The listing builds one solid part. Answer for the finished solid, in the listing's coordinates (mm). A direction names the side the tool comes from. Give positions to 0.01 mm unless a question says otherwise; leave off trailing zeros. Order: outer loops, then holes, each group sorted by start corner. A loop starts at its lowest first (then second) coordinate and runs counter-clockwise, first axis right, second up. Notation, with made-up numbers: (-39, -36.5) - (-24, -36.5) arc R4 ccw to (-24, -30.5) - close; hole circle Ø11 at (88, 36.25). An arc over 180 degrees is marked (long way). Use a Markdown table: item, result. Add a question column.
1) Flat-ended cylindrical pins translate along their axes: pin 1 (4 mm diameter, centred on x = 182, z = -41.5, fed in from +Y); pin 2 (10.5 mm diameter, centred on y = 1, z = -3.5, fed in from -X); pin 3 (1 mm diameter, centred on x = 128, y = 26, fed in from -Z); pin 4 (10 mm diameter, centred on x = 170, y = 12, fed in from -Z). Find the tip coordinate at first contact, or state that the pin passes through.
2) Straight lines are drawn through the part: line 1 (X direction, y = 0.5, z = -5); line 2 (X direction, y = 8, z = -32.5); line 3 (Y direction, x = 50.5, z = -25). For each, find the intervals that lie inside material, in ascending order.
3) For faces 1 (the face through (55, 4, -4)), 2 (the face through (94.33, 14.79, -55.07)), 3 (the face through (148, 30, -10)), determine the directions among +Z, -Z, +X, -X, +Y, -Y from which every point of the face is accessible in a straight line to the end or side of a thin tool.
4) The mould has two halves that part along X. Classify faces 4 (the face through (150.07, 10.872, -4.832)), 5 (the face through (0, 13, -30)), 6 (the face through (149, 0, -41)), 7 (the face through (148, 17, 0)): released by +X, released by -X, zero draft, split by the parting line, or undercut.
5) Find section D-D, the plane z = -14. Determine the outline of the cut face in (x, y).
6) Find section B-B, the plane x = 50. Determine the outline of the cut face in (y, z), plus the area to 3 significant figures.
7) Find section C-C, the plane z = -43. Determine the outline of the cut face in (x, y).
8) Find section A-A, the plane y = 22. Determine the outline of the cut face in (x, z), plus the area to 3 significant figures.
from build123d import *

# Parameters (mm, degrees)
BOSS_EXTRU_1_DEPTH         = 30
ESQUISSE2_W                = 300
ESQUISSE2_H                = 60
BOSS_EXTRU_2_DEPTH         = 5
ESQUISSE3_W                = 10
ESQUISSE3_H                = 5.78
ENL_V_MAT_EXTRU_3_DEPTH    = 14.49
ESQUISSE5_W                = 10
ESQUISSE5_H                = 17.8
ENL_V_MAT_EXTRU_5_DEPTH    = 5
BOSS_EXTRU_4_REACH         = 256.018
ENL_V_MAT_EXTRU_6_DEPTH    = 10
R_P_TITION_LIN_AIRE1_COUNT = 3
R_P_TITION_LIN_AIRE1_PITCH = 100


with BuildPart() as part:
    # Esquisse1 → Boss.-Extru.1 (new body)
    with BuildSketch(Plane(origin=(0, 0, 0), x_dir=(1, 0, 0), z_dir=(0, 1, 0))):
        with BuildLine():
            Line((0, 0), (300, 0))
            Line((300, 0), (300, 60))
            Line((300, 60), (288.5, 50))
            ThreePointArc((288.5, 50), (250, 11.5), (211.5, 50))
            Line((211.5, 50), (200, 60))
            Line((200, 60), (188.5, 50))
            ThreePointArc((188.5, 50), (150, 11.5), (111.5, 50))
            Line((111.5, 50), (100, 60))
            Line((100, 60), (88.5, 50))
            ThreePointArc((88.5, 50), (50, 11.5), (11.5, 50))
            Line((11.5, 50), (0, 60))
            Line((0, 60), (0, 0))
        make_face()
    extrude(amount=BOSS_EXTRU_1_DEPTH)

    # Esquisse2 → Boss.-Extru.2 (add)
    with BuildSketch(Plane.XZ):
        with Locations((150, -30)):
            Rectangle(ESQUISSE2_W, ESQUISSE2_H)
    extrude(amount=BOSS_EXTRU_2_DEPTH)

    # Esquisse3 → Enlèv. mat.-Extru.3 (cut, along a direction that is not the sketch's normal)
    with BuildSketch(Plane.XZ.offset(5)):
        with Locations((50, -2.89)):
            Rectangle(ESQUISSE3_W, ESQUISSE3_H)
        with Locations((250, -2.89)):
            Rectangle(ESQUISSE3_W, ESQUISSE3_H)
        with Locations((150, -2.89)):
            Rectangle(ESQUISSE3_W, ESQUISSE3_H)
    extrude(amount=-ENL_V_MAT_EXTRU_3_DEPTH, dir=(0, -0.96592582628907, 0.2588190451025146), mode=Mode.SUBTRACT)

    # Esquisse5 → Enlèv. mat.-Extru.5 (cut)
    with BuildSketch(Plane.XY):
        with Locations((250, 3.9)):
            Rectangle(ESQUISSE5_W, ESQUISSE5_H)
        with Locations((150, 3.9)):
            Rectangle(ESQUISSE5_W, ESQUISSE5_H)
        with Locations((50, 3.9)):
            Rectangle(ESQUISSE5_W, ESQUISSE5_H)
    extrude(amount=-ENL_V_MAT_EXTRU_5_DEPTH, mode=Mode.SUBTRACT)

    # Esquisse7 → Boss.-Extru.4 (add, up to next)
    with BuildSketch(Plane.ZY.offset(-55), mode=Mode.PRIVATE) as boss_extru_4_sk1:
        Polygon((-9.530287964, 8.996265223), (0, 12.8), (-9.530287964, 12.8), align=None)
    boss_extru_4_tool1 = extrude(boss_extru_4_sk1.sketch, amount=BOSS_EXTRU_4_REACH, mode=Mode.PRIVATE) - part.part
    boss_extru_4 = boss_extru_4_tool1.solids().sort_by_distance((55, 11.532088, -6.353525))[0]
    add(boss_extru_4)

    # Esquisse8 → Enlèv. mat.-Extru.6 (cut)
    with BuildSketch(Plane.ZY.offset(-55)):
        Polygon((-9.530287964, 8.996265223), (0, 12.8), (0, -5), (-5.78, -5), align=None)
    enl_v_mat_extru_6 = extrude(amount=ENL_V_MAT_EXTRU_6_DEPTH, mode=Mode.SUBTRACT)

    # Répétition linéaire1: Boss.-Extru.4, Enlèv. mat.-Extru.6 ×3
    with Locations(*[(i * R_P_TITION_LIN_AIRE1_PITCH, 0, 0) for i in range(1, R_P_TITION_LIN_AIRE1_COUNT)]):
        add(boss_extru_4)
        add(enl_v_mat_extru_6, mode=Mode.SUBTRACT)


solid = part.part
The answers:
| question | item | result |
|---|---|---|
| 1 | pin 1 | y = 0 |
| 1 | pin 2 | x = 0 |
| 1 | pin 3 | z = -18.76 |
| 1 | pin 4 | z = -20.72 |
| 2 | line 1 | 0 to 45, 55 to 145, 155 to 245, 255 to 300 |
| 2 | line 2 | 0 to 15.71, 84.29 to 115.71, 184.29 to 215.71, 284.29 to 300 |
| 2 | line 3 | -5 to 0 |
| 3 | face 1 | +Z |
| 3 | face 2 | -Z, +Y |
| 3 | face 3 | +Z, -Z, +X, -X, +Y |
| 4 | face 4 | undercut |
| 4 | face 5 | released by -X |
| 4 | face 6 | undercut |
| 4 | face 7 | zero draft |
| 5 | outline | (0, -5) - (300, -5) - (300, 30) - (263.65, 30) - (263.65, 0) - (236.35, 0) - (236.35, 30) - (163.65, 30) - (163.65, 0) - (136.35, 0) - (136.35, 30) - (63.65, 30) - (63.65, 0) - (36.35, 0) - (36.35, 30) - (0, 30) - close |
| 6 | outline | (-5, -60) - (0, -60) - (0, -11.5) - (30, -11.5) - (30, 0) - (12.8, 0) - (9, -9.53) - (-5, -5.78) - close |
| 6 | area | 520 mm2 |
| 7 | outline | (0, -5) - (300, -5) - (300, 30) - (287.86, 30) - (287.86, 0) - (212.14, 0) - (212.14, 30) - (187.86, 30) - (187.86, 0) - (112.14, 0) - (112.14, 30) - (87.86, 30) - (87.86, 0) - (12.14, 0) - (12.14, 30) - (0, 30) - close |
| 8 | outline | (0, -60) - (11.5, -50) arc R38.5 cw to (88.5, -50) - (100, -60) - (111.5, -50) arc R38.5 cw to (188.5, -50) - (200, -60) - (211.5, -50) arc R38.5 cw to (288.5, -50) - (300, -60) - (300, 0) - (0, 0) - close |
| 8 | area | 8,360 mm2 |
